Source: three-view drawing plus pictorial views. Frame: mm from the lowest corner of the part. Give positions to 0.01 mm unless a question says otherwise; leave off trailing zeros. Loops run counter-clockwise (first coordinate to the right, second up) from the corner with the lowest first, then second, coordinate; pieces in that order, holes last. Notation, with made-up numbers: (65, -24.5) -> (118, -24.5) arc R21 cw to (118, 9.5) -> close; hole circle Ø7 at (-9.75, -26.5). An arc over 180 degrees is marked (long way). Answer as a JSON object with one key per item and string values. Group by question number.
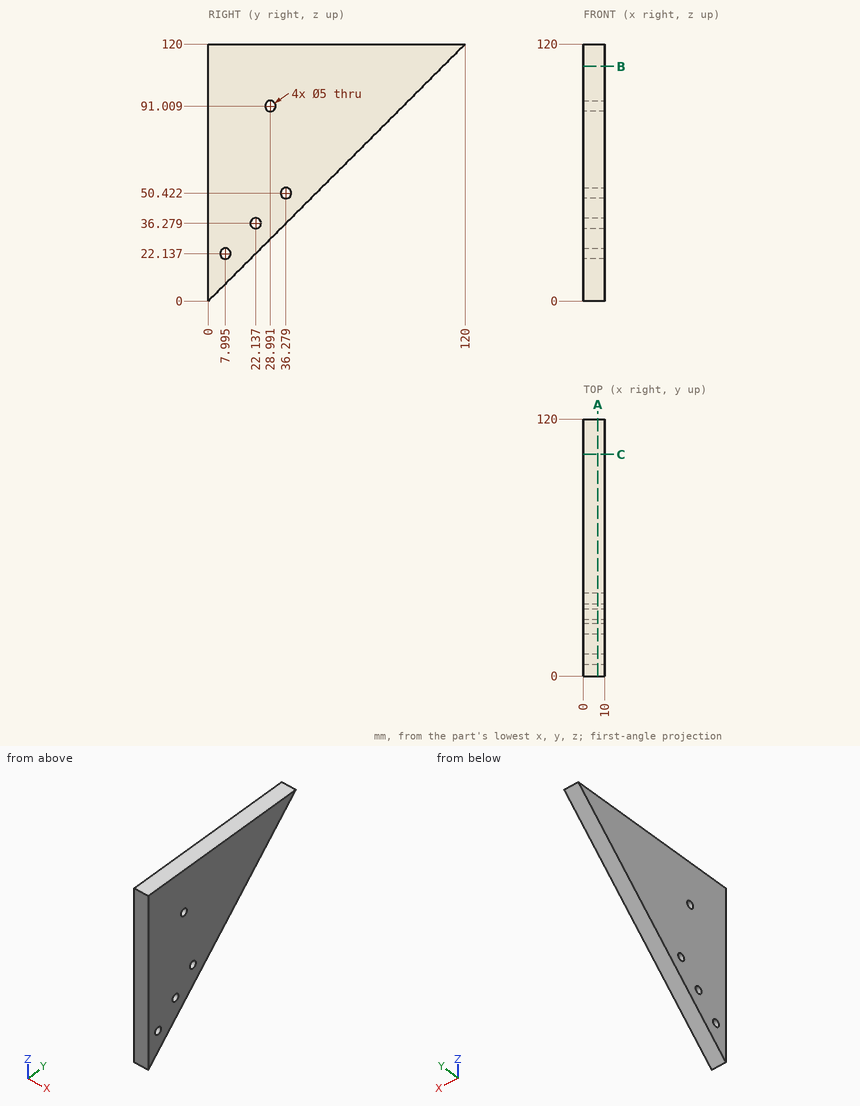
Q1. Ray query, probe 1 along Y at (x, z) = (6.75, 48.5); probe 2 along Y at (x, z) = (5.5, 36.5) (1 decimal); probe 3 along Y at (x, z) = (3.25, 75). Return the intervals inside material, ascending.
Q2. Section B-B on z = 109.5. Return the cut outline in (x, y), then the cut area to 4 significant figures.
Q3. Section A-A on x = 6.75. Return the cut outline in (y, z) (1 decimal), then the cut area to 3 significant figures.
Q4. Pin query (flat end, axial travel): pin 1 Ø4.5 at (y, z) = (22.14, 36.28) entering from -X; pin 2 Ø5 at (x, z) = (6, 35) entering from +Y; pin 3 Ø6 at (x, y) = (7.5, 66.5) entering from -Z. Return the tip coordinate at first contact, or that it passes through.
Q5. Section C-C on y = 103.5. Return the cut outline in (x, z).
Numbers:
{
 "1": {"probe 1": "y = 0 to 34.68, 37.88 to 48.5", "probe 2": "y = 0 to 19.6, 24.6 to 36.5", "probe 3": "y = 0 to 75"},
 "2": {"outline": "(0, 0) -> (10, 0) -> (10, 109.5) -> (0, 109.5) -> close", "area": "1,095 mm²"},
 "3": {"outline": "(0, 0) -> (120, 120) -> (0, 120) -> close; hole circle Ø5 at (8, 22.1); hole circle Ø5 at (22.1, 36.3); hole circle Ø5 at (29, 91); hole circle Ø5 at (36.3, 50.4)", "area": "7,120 mm²"},
 "4": {"pin 1": "passes through", "pin 2": "stops at y = 37.5", "pin 3": "stops at z = 63.5"},
 "5": {"outline": "(0, 103.5) -> (10, 103.5) -> (10, 120) -> (0, 120) -> close"}
}
